The model under review builds one solid part; all positions refer to its coordinate system, in mm. A direction names the side the tool comes from. Round coordinates to 2 decimals unless told otherwise and drop trailing zeros. Loops run counter-clockwise (first coordinate to the right, second up) from the corner with the lowest first, then second, coordinate; pieces in that order, holes last. Notation, with made-up numbers: (-39.5, -16.5) -> (-7.5, -16.5) arc R22 ccw to (-7.5, -7.5) -> close; hole circle Ø8 at (77.25, -18.5). An arc over 180 degrees is marked (long way). Write each question's results on one line, items separated by ' | '. Start each with the question number.
Item 1: Tool access review of faces 5 (the cylindrical face through (-31.51, -7.1, 2.86)), 6 (the flat face through (-2, 0, 0.9)), 7 (the cylindrical face through (-0.65, 16.93, 1.73)): name each direction out of +Z, -Z, +X, -X, +Y, -Y from which nothing blocks a thin tool from reaching the whole face with its end or side.
Item 2: We need section A-A (x = 0). Give the boundary of the cut face in (y, z).
Item 3: We need section C-C (z = 4.35). Give the number of separate pieces and of enclosed holes in the cut face, and give its area (3 significant figures).
Item 4: Clearance check with flat-ended pins moving along their axes: pin 1 Ø1.8 at (x, y) = (-1.5, 13.5) entering from -Z; pin 2 Ø0.8 at (x, y) = (-31.5, -2.5) entering from +Z; pin 3 Ø9.5 at (x, y) = (28, 14) entering from -Z; pin 4 Ø11 at (x, y) = (1, 0.5) entering from +Z. State where each tip first meets the part, or that it passes through.
Item 5: For L1, parallel to X at y = 14, z = 0.8; L2, parallel to Y at x = 28, z = 4.5; L3, parallel to Y at x = -28, z = 4.5, list the stretches that pass through material, from the lowest coordinate up. Write a range as from..to.
Item 6: Mouldability with a two-part tool opening along Y and no side actions: class faces 1 (the cylindrical face through (-0.65, -11.07, 1.73)), 2 (the cylindrical face through (-30.797, 16.859, 2.535)), 3 (the flat face through (0, 12, 5)), 4 (the flat face through (-1.3, 12.7, 3.5)) as pulls with the +Y half, pulls with the -Y half, needs draft (parallel to the pull), parting line crosses it, or undercut.
Solid Edge part; units mm, degrees
sketch "Sketch1" plane through (0, 0, 0) normal (0, 0, 1) x (1, 0, 0)
  line L0 (32, -18) -> (32, 18)
  line L1 (32, 18) -> (-32, 18)
  line L2 (-32, 18) -> (-32, -18)
  line L3 (-32, -18) -> (32, -18)
extrude "Protrusion1" add sketch "Sketch1" along normal blind 5
sketch "Sketch2" plane through (-32, 0, 2.5) normal (-1, 0, 0) x (0, -1, 0)
  line L0 (-5, -0.5) -> (5, -0.5)
  line L1 (-8, 2.5) -> (8, 2.5)
  arc A0 (8, 2.5) -> (5, -0.5) centre (5, 2.5) cw
  arc A1 (-5, -0.5) -> (-8, 2.5) centre (-5, 2.5) cw
extrude "VaciadoExtruido_2" cut sketch "Sketch2" against normal blind 1
sketch "Sketch3" plane through (-31, 0, 2.5) normal (-1, 0, 0) x (0, -1, 0)
  line L0 (-5, -1.6) -> (5, -1.6)
  line L1 (-9.1, 2.5) -> (9.1, 2.5)
  arc A0 (9.1, 2.5) -> (5, -1.6) centre (5, 2.5) cw
  arc A1 (-5, -1.6) -> (-9.1, 2.5) centre (-5, 2.5) cw
extrude "VaciadoExtruido_3" cut sketch "Sketch3" against normal blind 62
fillet "Redondeo_3" radius 4.1 3 edges at (31, 7.8991, 2.1009) (31, -7.8991, 2.1009) (31, 0, 0.9)
sketch "Sketch4" plane through (0, 0, 5) normal (0, 0, 1) x (1, 0, 0)
  circle A0 centre (-28, 14) radius 1.6
extrude "Cutout1" cut sketch "Sketch4" against normal through all
sketch "Sketch5" plane through (0, 0, 0) normal (0, 0, -1) x (1, 0, 0)
  circle A0 centre (-28, -14) radius 3
extrude "VaciadoExtruido_5" cut sketch "Sketch5" against normal blind 3.5
pattern_linear "Pattern1" count 3 spacing 28 along (1, 0, 0) count 2 spacing 28 along (0, -1, 0) of "VaciadoExtruido_5", "Cutout1"
fillet "Redondeo_4" radius 4 4 edges at (-32, 18, 2.5) (-32, -18, 2.5) (32, 18, 2.5) (32, -18, 2.5)
Here are the results:
1) face 5: +Z, -X | face 6: +Z | face 7: -Z
2) outline: (-18, 0) -> (-17, 0) -> (-17, 3.5) -> (-15.6, 3.5) -> (-15.6, 5) -> (-18, 5) -> close; (-12.4, 3.5) -> (-11, 3.5) -> (-11, 0) -> (11, 0) -> (11, 3.5) -> (12.4, 3.5) -> (12.4, 5) -> (9.1, 5) arc R4.1 cw to (5, 0.9) -> (-5, 0.9) arc R4.1 cw to (-9.1, 5) -> (-12.4, 5) -> close; (15.6, 3.5) -> (17, 3.5) -> (17, 0) -> (18, 0) -> (18, 5) -> (15.6, 5) -> close
3) separate pieces: 1 | enclosed holes: 6 | area: 1,110 mm2
4) pin 1: stops at z = 3.5 | pin 2: stops at z = 2 | pin 3: stops at z = 0 | pin 4: stops at z = 1.02
5) L1: x = -32..-31, -25..-3, 3..25, 31..32 | L2: y = -18..-15.6, -12.4..-8.92, 8.92..12.4, 15.6..18 | L3: y = -18..-15.6, -12.4..-9.07, 9.07..12.4, 15.6..18
6) face 1: undercut | face 2: pulls with the +Y half | face 3: needs draft | face 4: undercut
